Read the model definition and answer for the solid it produces. Units are mm, in the model's axes. A direction names the side the tool comes from. Coordinates: 2 decimals unless noted, no trailing zeros. Loops run counter-clockwise (first coordinate to the right, second up) from the corner with the lowest first, then second, coordinate; pieces in that order, holes last. Notation, with made-up numbers: (-25.75, -36) - (-7.75, -36) arc R9 ccw to (-7.75, -30) - close; hole circle Ø9 at (86.25, -29). An arc over 180 degrees is marked (long way). Use one line per item in the form item = value.
from build123d import *

# Parameters (mm, degrees)
F3_R          = 0.5
F4_W          = 2
F4_H          = 6
F5_DEPTH      = 5
F5_DEPTH_BACK = 1
F6_R          = 1


with BuildPart() as f2:
    # F2: sweep along a path in F0
    with BuildLine(Plane.XZ) as f2_path:
        Line((0, 0), (2, 0))
        ThreePointArc((2, 0), (3.4142135624, 0.5857864376), (4, 2))
        Line((4, 2), (4, 3))
    # F1 (on Right) → F2 (sweep)
    with BuildSketch(Plane.YZ):
        with BuildLine():
            Line((1, -1), (1, 0))
            ThreePointArc((1, 0), (0, 1), (-1, 0))
            Line((-1, 0), (-1, -1))
            Line((-1, -1), (1, -1))
        make_face()
    sweep(path=f2_path.line)

    # F3
    f3_edges = [f2.edges().sort_by_distance(p)[0] for p in [
        (5, 0, 3),
        (3, 0, 3),
        (4.12132, -1, -0.12132),
        (4.12132, 1, -0.12132),
    ]]
    fillet(f3_edges, radius=F3_R)

    # F4 (on Top) → F5 (join, two sides)
    with BuildSketch(Plane.XY) as f5_sk:
        with Locations((-1, 0)):
            Rectangle(F4_W, F4_H)
    extrude(amount=F5_DEPTH)
    extrude(f5_sk.sketch, amount=-F5_DEPTH_BACK)

    # F6
    f6_edges = [f2.edges().sort_by_distance(p)[0] for p in [
        (-1, -3, -1),
        (-1, -3, 5),
        (-1, 3, 5),
        (-1, 3, -1),
    ]]
    fillet(f6_edges, radius=F6_R)


solid = f2.part
Item 1: For a pull along X with two mould halves and no side action, classify faces 4 (the cylindrical face through (3, 0, 2.3)), 5 (the flat face through (-2, 0, 2)), 6 (the cylindrical face through (-0.986, -2.699, 4.715)), 7 (the cylindrical face through (4.1, 0.01, -0.14)) as +X half, -X half, draft (parallel to the pull), parting line (faces both ways), or undercut.
Results below:
face_4 = undercut
face_5 = -X half
face_6 = draft
face_7 = +X half
Item 2: The part is cut by section C-C on x = 0.75. Give the vertices of the cut face in (y, z), plus the area to 3 significant figures.
Results below:
outline = (-1, -0.5) arc R0.5 ccw to (-0.5, -1) - (0.5, -1) arc R0.5 ccw to (1, -0.5) - (1, 0) arc R1 ccw to (-1, 0) - close
area = 3.46 mm²
Item 3: The part is cut by section D-D on z = 4.45. Give the vertices of the cut face in (x, y).
Results below:
outline = (-2, -2.89) - (0, -2.89) - (0, 2.89) - (-2, 2.89) - close
Item 4: The part is cut by section A-A on x = -1.25. Give the vertices of the cut face in (y, z), plus the area to 3 significant figures.
Results below:
outline = (-3, 0) arc R1 ccw to (-2, -1) - (2, -1) arc R1 ccw to (3, 0) - (3, 4) arc R1 ccw to (2, 5) - (-2, 5) arc R1 ccw to (-3, 4) - close
area = 35.1 mm²
Item 5: Find the intervals of material crossed by L1, parallel to X at y = 2, z = -0.15; L2, parallel to Y at x = 0.75, z = 0.05; L3, parallel to Z at x = 3.5, y = -0.7, in increasing order.
Results below:
L1 = -2 to 0
L2 = -1 to 1
L3 = -0.55 to 2.85
Item 6: Each of these flat-tipped pins is pushed along its axis until it touches: P1, Ø1.5, axis at x = 2.5, y = 0.5, coming from the +Z side; P2, Ø2.5, axis at x = 2, z = 1.5, coming from the +Y side; P3, Ø3, axis at x = 3.5, y = -2, coming from the +Z side. Where does it stop, or does it pass through?
Results below:
P1 = 2.87
P2 = 0.97
P3 = 3
Item 7: Which of the six approach directions +Z, -Z, +X, -X, +Y, -Y give full straight-line access (tool end or side, diameter ignored) to faces 1 (the flat face through (3, 1, 0)), 2 (the flat face through (3, -1, 0)), 3 (the flat face through (4, 0, 3))?
Results below:
face_1 = +Z, -Z, +X, +Y
face_2 = +Z, -Z, +X, -Y
face_3 = +Z, +X, +Y, -Y
Item 8: The part is cut by section B-B on y = -1.45. Give the vertices of the cut face in (x, z).
Results below:
outline = (-2, -1) - (0, -1) - (0, 5) - (-2, 5) - close
